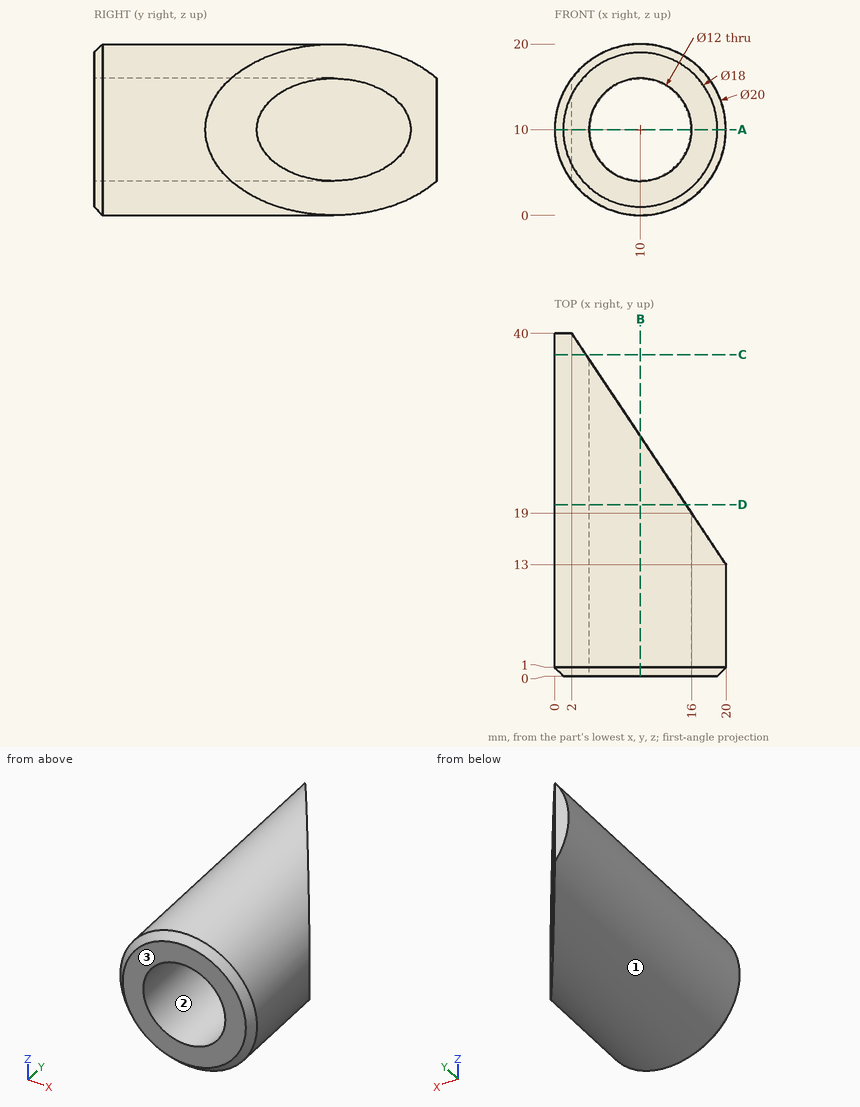
Answer from the drawing. Dimensions are ordinates in mm from the lowest x, y and z of the part. Coordinates: 2 decimals unless noted, no trailing zeros. Loops run counter-clockwise (first coordinate to the right, second up) from the corner with the lowest first, then second, coordinate; pieces in that order, holes last. Notation, with made-up numbers: (-39, 61) -> (9, 61) arc R33 ccw to (9, 95) -> close; hole circle Ø2 at (-4.5, 19.5). An arc over 180 degrees is marked (long way). Return JSON: item names as keys, results as strings.
Item 1: Find section A-A (z = 10). Determine the outline of the cut face in (x, y), plus the area to 3 significant figures.
Answers:
{"outline": "(0, 1) -> (1, 0) -> (4, 0) -> (4, 37) -> (2, 40) -> (0, 40) -> close; (16, 0) -> (19, 0) -> (20, 1) -> (20, 13) -> (16, 19) -> close", "area": "220 mm2"}
Item 2: Flat-ended cylindrical pins translate along their axes: P1, Ø4, axis at x = 2.5, y = 26, coming from the +Z side; P2, Ø3, axis at x = 5.5, y = 5, coming from the -Z side; P3, Ø6, axis at x = 15.5, y = 23, coming from the -Z side; P4, Ø11, axis at x = 10, z = 10, coming from the -Y side. Find the tip coordinate at first contact, or state that the pin passes through.
Answers:
{"P1": "stops at z = 18.35", "P2": "stops at z = 0.46", "P3": "stops at z = 0.32", "P4": "passes through"}
Item 3: For a pull along X with two mould halves and no side action, classify the marked faces 1, 2 and 3 as +X half, -X half, draft (parallel to the pull), parting line (faces both ways), or undercut.
Answers:
{"face 1": "parting line", "face 2": "undercut", "face 3": "draft"}
Item 4: Find section B-B (x = 10). Determine the outline of the cut face in (y, z).
Answers:
{"outline": "(0, 1) -> (1, 0) -> (28, 0) -> (28, 4) -> (0, 4) -> close; (0, 16) -> (28, 16) -> (28, 20) -> (1, 20) -> (0, 19) -> close"}
Item 5: Find section D-D (y = 20). Determine the outline of the cut face in (x, z).
Answers:
{"outline": "(15.33, 1.54) -> (15.33, 7.25) arc R6 cw (long way) to (15.33, 12.75) -> (15.33, 18.46) arc R10 ccw (long way) to start"}
Item 6: Find section C-C (y = 37.5). Determine the outline of the cut face in (x, z).
Answers:
{"outline": "(3.67, 2.26) -> (3.67, 17.74) arc R10 ccw to start"}
Item 7: Find the intervals of material crossed by probe 1 along Z at (x, y) = (10, 10); probe 2 along X at (y, z) = (22.5, 10), in increasing order.
Answers:
{"probe 1": "z = 0 to 4, 16 to 20", "probe 2": "x = 0 to 4"}
